Could you check a few things on this drawing? It's one solid part, dimensions in mm from its lowest x, y, z. A direction names the side the tool comes from. Give positions to 0.01 mm unless a question says otherwise; leave off trailing zeros. Loops run counter-clockwise (first coordinate to the right, second up) from the corner with the lowest first, then second, coordinate; pieces in that order, holes last. Notation, with made-up numbers: M -15.75,15.5 L 14.25,15.5 A13 cw 14.25,25.5 Z; hole C 71.5,-10.5 d7. An arc over 180 degrees is marked long. One line per item, written item: value. Start each with the question number.
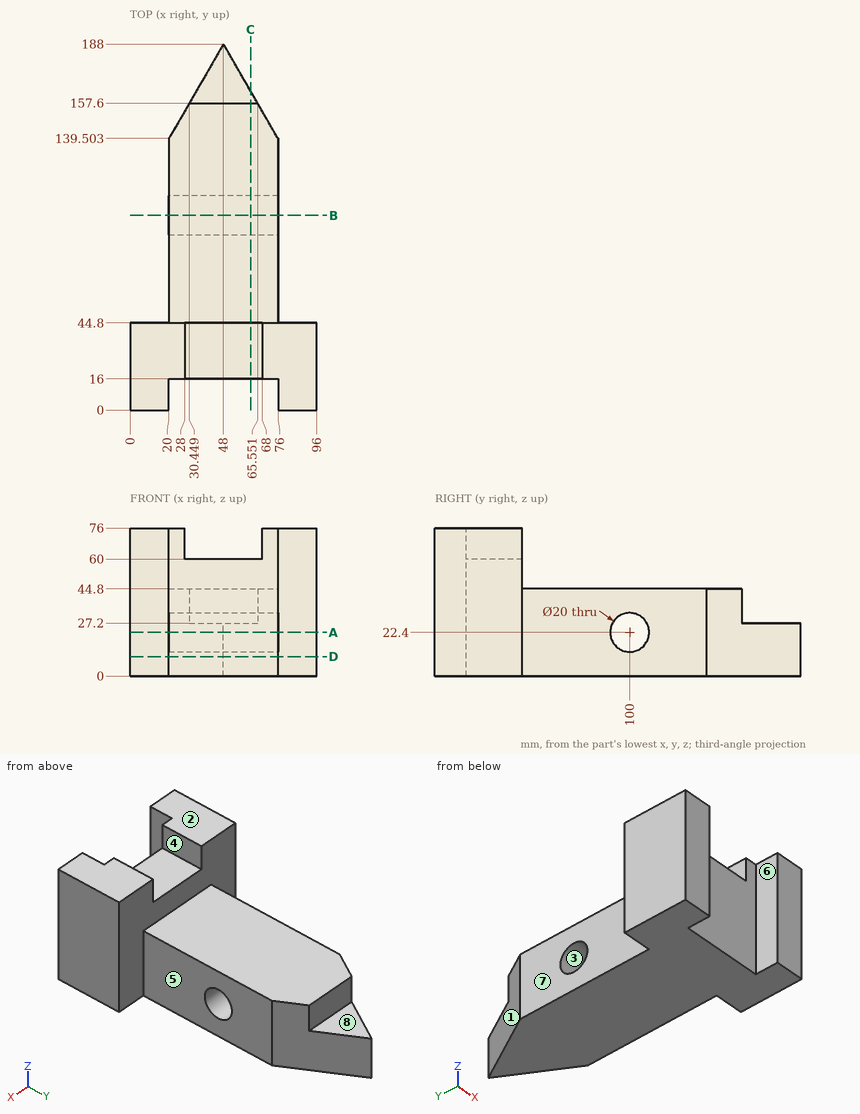
Q1. If we section it at A-A, the plane z = 22.4: Write out the boundary of the cut face in (x, y).
Q2. For P1, Ø17, axis at x = 35.5, z = 54, coming from the -Y side; P2, Ø4, axis at x = 27.5, z = 18.5, coming from the +Y side (1 decimal); P3, Ø5.5, axis at x = 48.5, z = 39, coming from the +Y side, each with a flat end and sliding along its axis, tell me the tip position at first contact or that it passes through.
Q3. If we section it at D-D, the plane z = 10: Write out the boundary of the cut face in (x, y), plus the area to 3 significant figures.
Q4. Which directions (+Z, -Z, +X, -X, +Y, -Y) give clear straight access to the entire face, cutting with the end or side of a thin tool? Please do the marked faces 4, 5, 6, 7 and 8.
Q5. If we section it at C-C, the plane x = 62: Write out the boundary of the cut face in (y, z).
Q6. If we mould it in two halves opening along Z, with no side actions, what happens to the marked faces 1, 2 and 3? For each: released by +Z, released by -Z, zero draft, split by the parting line, or undercut.
Q7. I need wall thicknesses on line 1 along X through (y, z) = (22, 62); line 2 along Z through (x, y) = (46.5, 100); line 3 along X through (y, z) = (8.5, 27.5). Which ranges of each line are inside material? Lowest first, please.
Q8. If we section it at B-B, the plane y = 100: Write out the boundary of the cut face in (x, z).
Response:
1. outline: M 0,0 L 20,0 L 20,16 L 76,16 L 76,0 L 96,0 L 96,44.8 L 76,44.8 L 76,90 L 20,90 L 20,44.8 L 0,44.8 Z; M 20,110 L 76,110 L 76,139.5 L 48,188 L 20,139.5 Z
2. P1: y = 16
2. P2: y = 156
2. P3: y = 157.6
3. outline: M 0,0 L 20,0 L 20,16 L 76,16 L 76,0 L 96,0 L 96,44.8 L 76,44.8 L 76,139.5 L 48,188 L 20,139.5 L 20,44.8 L 0,44.8 Z
3. area: 10,100 mm^2
4. face 4: +Z, +Y, -Y
4. face 5: +Z, -Z, +X, +Y
4. face 6: +Z, -Z, -Y
4. face 7: +Z, -Z, -X, +Y
4. face 8: +Z, +X, -X, +Y
5. outline: M 16,0 L 163.75,0 L 163.75,27.2 L 157.6,27.2 L 157.6,44.8 L 44.8,44.8 L 44.8,60 L 16,60 Z; hole C 100,22.4 d20
6. face 1: zero draft
6. face 2: released by +Z
6. face 3: undercut
7. line 1: 0 to 28, 68 to 96
7. line 2: 0 to 12.4, 32.4 to 44.8
7. line 3: 0 to 20, 76 to 96
8. outline: M 20,0 L 76,0 L 76,12.4 L 20,12.4 Z; M 20,32.4 L 76,32.4 L 76,44.8 L 20,44.8 Z
